The drawing under review shows one solid part. Ordinate dimensions are in mm from its lowest x, y, z. A direction names the side the tool comes from. Give positions to 0.01 mm unless a question says otherwise; leave off trailing zeros. Write each loop counter-clockwise with the first axis right and the second up, starting at its lowest first coordinate (ties: lowest second). Pieces come first, ordered by that corner, then holes. Notation, with made-up numbers: M -39,64.5 L 16,64.5 A19 ccw 16,89.5 Z; hole C 31,-29 d5. An arc over 180 degrees is marked long. One line per item, written item: value. Start each with the question number.
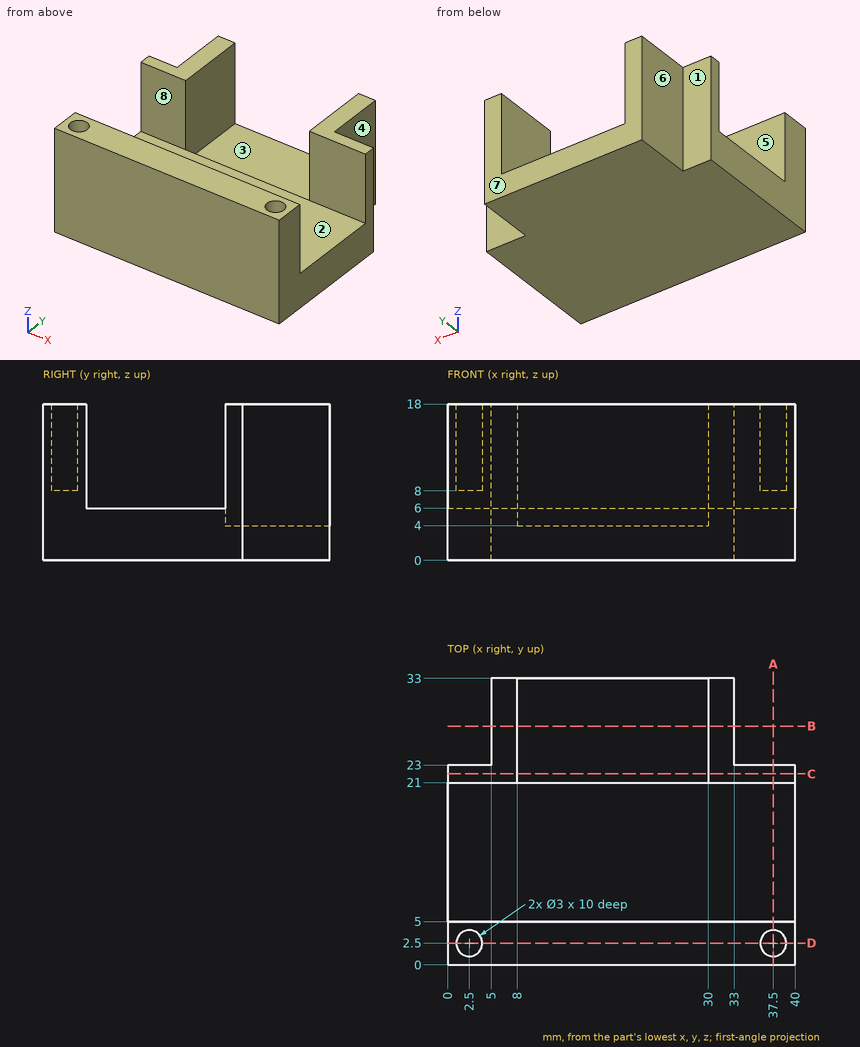
Q1. Machinability: for the marked faces 1, 2, 3 and 4, which of the approach directions +Z, -Z, +X, -X, +Y, -Y give a long, thin tool a straight path to every point of the face, cutting with its end or side? Answer none if there is none.
Q2. Wall thickness on line 1 (Y direction, x = 2.5, z = 10.5); line 2 (X direction, y = 24.5, z = 6.75); line 3 (Y direction, x = 5.5, z = 10): over which ranges is each line inside the solid? List them lowest first. Write a range as from..to.
Q3. Take a section at A-A, the plane x = 37.5. Give the boundary of the cut face in (y, z).
Q4. For P1, Ø1.5, axis at x = 26.5, y = 20, coming from the -Z side; P2, Ø5, axis at x = 13, y = 12.5, coming from the +Z side; P3, Ø9.5, axis at y = 29, z = 10.5, coming from the +X side; P4, Ø1.5, axis at x = 2, z = 6, coming from the +Y side, all flat-tipped, find the tip position at first contact; note any pin that passes through.
Q5. Take a section at D-D, the plane y = 2.5. Give the boundary of the cut face in (x, z), then the cut area to 3 significant figures.
Q6. Take a section at B-B, the plane y = 27.5. Give the boundary of the cut face in (x, z), then the cut area to 3 significant figures.
Q7. The part is to be moulded in two halves that separate along Y. For the marked faces 5, 6, 7 and 8, say which applies: pulls with the +Y half, pulls with the -Y half, needs draft (parallel to the pull), parting line crosses it, or undercut.
Q8. Take a section at C-C, the plane y = 22. Give the boundary of the cut face in (x, z).
Results list:
1. face 1: +Z, -Z, -X, +Y
1. face 2: +Z, +X, -X
1. face 3: +Z, +Y
1. face 4: +Z, -Z, +X, +Y
2. line 1: y = 0..1, 4..5, 21..23
2. line 2: x = 5..8, 30..33
2. line 3: y = 0..5, 21..33
3. outline: M 0,0 L 23,0 L 23,18 L 21,18 L 21,6 L 5,6 L 5,18 L 4,18 L 4,8 L 1,8 L 1,18 L 0,18 Z
4. P1: stops at z = 0
4. P2: stops at z = 6
4. P3: stops at x = 33
4. P4: stops at y = 23
5. outline: M 0,0 L 40,0 L 40,18 L 39,18 L 39,8 L 36,8 L 36,18 L 4,18 L 4,8 L 1,8 L 1,18 L 0,18 Z
5. area: 660 mm^2
6. outline: M 5,0 L 33,0 L 33,18 L 30,18 L 30,4 L 8,4 L 8,18 L 5,18 Z
6. area: 196 mm^2
7. face 5: undercut
7. face 6: needs draft
7. face 7: pulls with the +Y half
7. face 8: undercut
8. outline: M 0,0 L 40,0 L 40,18 L 30,18 L 30,4 L 8,4 L 8,18 L 0,18 Z
